For this review, use the dimensioned drawing (mm, ordinates from the lowest corner) and the shaded views. Coordinates: 2 decimals unless noted, no trailing zeros. Loops run counter-clockwise (first coordinate to the right, second up) from the corner with the lowest first, then second, coordinate; pieces in that order, holes last. Notation, with made-up numbers: M 29,-7.75 L 73,-7.75 A25 ccw 73,10.25 Z; hole C 21,60.5 d8. An arc over 180 degrees is marked long. Write item = value, one per line.
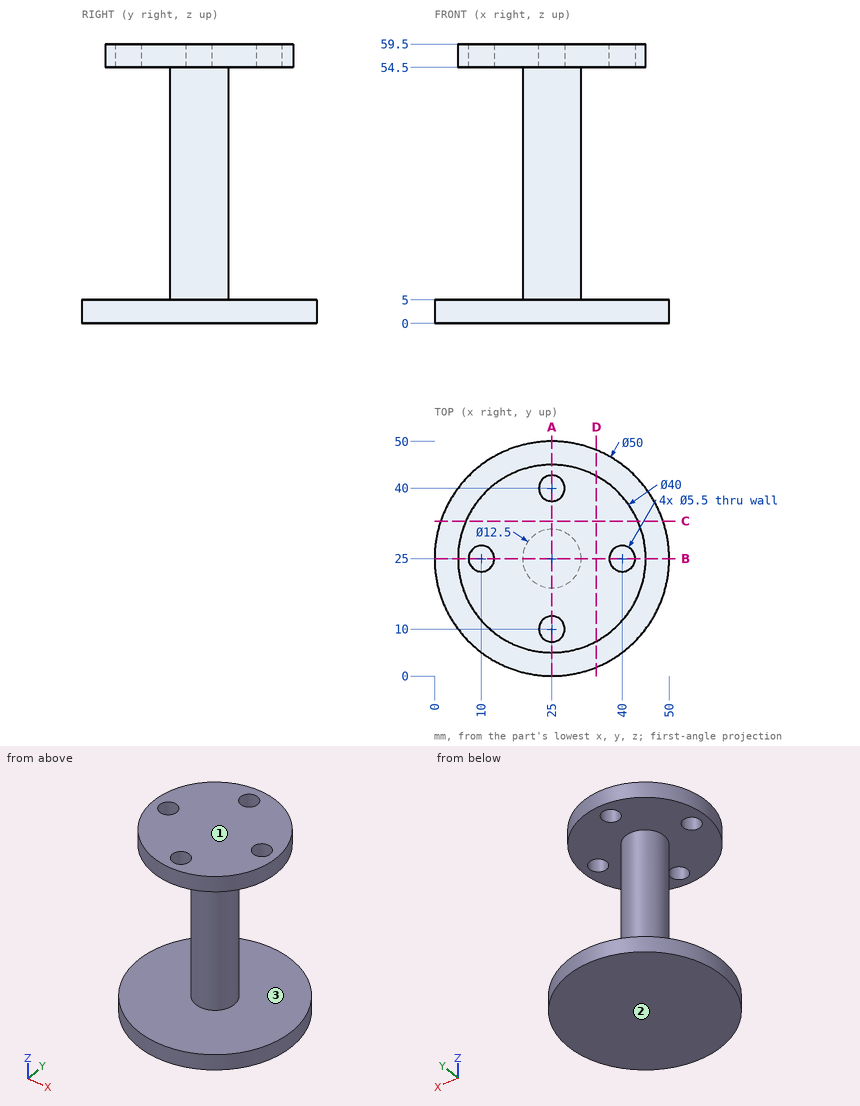
Q1. Add section A-A (x = 25). Write out the cut boundary in (y, z), and give its area (3 significant figures).
Solved:
outline = M 0,0 L 50,0 L 50,5 L 31.25,5 L 31.25,54.5 L 37.25,54.5 L 37.25,59.5 L 12.75,59.5 L 12.75,54.5 L 18.75,54.5 L 18.75,5 L 0,5 Z; M 5,54.5 L 7.25,54.5 L 7.25,59.5 L 5,59.5 Z; M 42.75,54.5 L 45,54.5 L 45,59.5 L 42.75,59.5 Z
area = 1,010 mm²
Q2. Add section C-C (y = 33). Write out the cut boundary in (x, z).
Solved:
outline = M 1.31,0 L 48.69,0 L 48.69,5 L 1.31,5 Z; M 6.67,54.5 L 43.33,54.5 L 43.33,59.5 L 6.67,59.5 Z
Q3. Draft analysis for pull direction Z (two halves, no side actions). For the marked faces 1, 2 and 3, state which applies: +Z half, -Z half, draft (parallel to the pull), parting line (faces both ways), or undercut.
Solved:
face_1 = +Z half
face_2 = -Z half
face_3 = undercut
Q4. For pin 1 Ø3.5 at (x, y) = (25, 40) entering from +Z; pin 2 Ø6 at (y, z) = (27, 43) entering from +X, all flat-tipped, find the tip position at first contact; note any pin that passes through.
Solved:
pin_1 = 5
pin_2 = 31.25
Q5. For line 1 along Y through (x, z) = (25, 57.8); line 2 along Z through (x, y) = (35, 9.5); line 3 along Z through (x, y) = (41, 40), list the stretches that pass through material, from the lowest coordinate up.
Solved:
line_1 = 5 to 7.25, 12.75 to 37.25, 42.75 to 45
line_2 = 0 to 5, 54.5 to 59.5
line_3 = 0 to 5
Q6. Add section D-D (x = 34.5). Write out the cut boundary in (y, z), and give its area (3 significant figures).
Solved:
outline = M 1.88,0 L 48.12,0 L 48.12,5 L 1.88,5 Z; M 7.4,54.5 L 42.6,54.5 L 42.6,59.5 L 7.4,59.5 Z
area = 407 mm²
